Read the model definition and answer for the solid it produces. Units are mm, in the model's axes. A direction names the side the tool comes from. Give positions to 0.01 mm unless a question says otherwise; leave off trailing zeros. Write each loop counter-clockwise with the first axis right and the second up, starting at its lowest first coordinate (ties: lowest second). Pieces come first, ordered by that corner, then holes. Notation, with made-up numbers: (75.5, -23.5) - (86.5, -23.5) arc R16 ccw to (86.5, -0.5) - close; hole circle Ø11 at (55, 60.5). An arc over 180 degrees is marked (long way). Answer as a JSON object with one key per item and string values. Group by question number.
```python
from build123d import *

# Parameters (mm, degrees)
F0_W     = 119
F0_H     = 119
F1_DEPTH = 2.2
F3_DEPTH = 30
F4_R     = 38
F5_DEPTH = 30
F6_T     = -2.2
F7_DEPTH = 1


with BuildPart() as f1:
    # F0 (on Top) → F1 (new body)
    with BuildSketch(Plane.XY):
        Rectangle(F0_W, F0_H)
    extrude(amount=F1_DEPTH)

    # F7 (add): a face of the model
    f7_faces = [f1.faces().sort_by_distance(p)[0] for p in [
        (0, 0, 2.2),
    ]]


with BuildPart() as f3:
    # F2 (on face) → F3 (new body)
    with BuildSketch(Plane.XY.offset(2.2)):
        with BuildLine():
            ThreePointArc((-54.5, 0), (-40.3438347211, -41.7435124756), (0, -59.5))
            ThreePointArc((0, -59.5), (59.5, 0), (0, 59.5))
            Line((0, 59.5), (-59.5, 59.5))
            Line((-59.5, 59.5), (-59.5, 0))
            Line((-59.5, 0), (-54.5, 0))
        make_face()
    extrude(amount=F3_DEPTH)

    # F4 (on face) → F5 (cut, through all)
    with BuildSketch(Plane.XY.offset(32.2)):
        Circle(F4_R)
    extrude(amount=-F5_DEPTH, mode=Mode.SUBTRACT)

    # F6
    f6_openings = [f3.faces().sort_by_distance(p)[0] for p in [
        (-59.5, 29.75, 17.2),
    ]]
    offset(amount=F6_T, openings=f6_openings, kind=Kind.INTERSECTION)


with BuildPart() as f1_1:
    add(f1.part)

    add(f3.part)  # F7 merges F3
    extrude(f7_faces, amount=-F7_DEPTH)


solid = f1_1.part
```
1) Which of the six approach directions +Z, -Z, +X, -X, +Y, -Y give full straight-line access (tool end or side, diameter ignored) to faces 5 (the flat face through (-56, 2.2, 17)), 6 (the cylindrical face through (57.286, -1.26, 17.021)), 7 (the flat face through (45, 48, 2.2)), 8 (the flat face through (47, -47, 2.2)), 9 (the flat face through (-1, 1, 2.2))?
2) Find section D-D, the plane x = -15. Write down the section's boundary in (y, z), and give its area (3 significant figures).
3) For a pull along X with two mould halves and no side action, classify faces 1 (the cylindrical face through (-39.93, -38.89, 17.02)), 2 (the cylindrical face through (17.535, -33.713, 17.41)), 3 (the flat face through (-1, 1, 0)), 4 (the cylindrical face through (-40.77, -41.27, 16.99)) as released by +X, released by -X, zero draft, split by the parting line, or undercut.
4) Find section B-B, the plane x = 21.5. Write down the section's boundary in (y, z).
5) Flat-ended cylindrical pins translate along their axes: pin 1 Ø10 at (y, z) = (10.5, 10.5) entering from +X; pin 2 Ø3 at (y, z) = (-45, 9) entering from +X; pin 3 Ø2.5 at (x, z) = (-57.5, 10.5) entering from -Y. Find the tip coordinate at first contact, or state that the pin passes through.
6) Find the intervals of material crossed by line 1 (Z direction, x = 22, y = 39); line 2 (X direction, y = -6.5, z = 14.5); line 3 (Y direction, x = 12, z = 15), in increasing order. Write a range as [from, to].
7) Find section A-A, the plane z = 17. Write down the section's boundary in (x, y), and give its area (3 significant figures).
8) Find section C-C, the plane y = -42.5. Write down the section's boundary in (x, z), and give its area (3 significant figures).
Values follow:
{
 "1": {"face 5": "-X", "face 6": "none", "face 7": "+Z, +X, +Y", "face 8": "+Z, +X, -Y", "face 9": "+Z"},
 "2": {"outline": "(-59.5, 0) - (59.5, 0) - (59.5, 32.2) - (34.91, 32.2) - (34.91, 2.2) - (-34.91, 2.2) - (-34.91, 32.2) - (-57.4, 32.2) - (-57.4, 2.2) - (-59.5, 2.2) - close; hole (-55.11, 4.4) - (-37.3, 4.4) - (-37.3, 30) - (-55.11, 30) - close; hole (37.3, 4.4) - (57.3, 4.4) - (57.3, 30) - (37.3, 30) - close", "area": "706 mm2"},
 "3": {"face 1": "undercut", "face 2": "undercut", "face 3": "zero draft", "face 4": "released by -X"},
 "4": {"outline": "(-59.5, 0) - (59.5, 0) - (59.5, 2.2) - (55.48, 2.2) - (55.48, 32.2) - (31.33, 32.2) - (31.33, 2.2) - (-31.33, 2.2) - (-31.33, 32.2) - (-55.48, 32.2) - (-55.48, 2.2) - (-59.5, 2.2) - close; hole (-53.11, 4.4) - (-33.97, 4.4) - (-33.97, 30) - (-53.11, 30) - close; hole (33.97, 4.4) - (53.11, 4.4) - (53.11, 30) - (33.97, 30) - close"},
 "5": {"pin 1": "stops at x = 59.25", "pin 2": "stops at x = 40.6", "pin 3": "stops at y = 0"},
 "6": {"line 1": "z = [0, 4.4], [30, 32.2]", "line 2": "x = [-54.68, -52.48], [-39.67, -37.44], [37.44, 39.67], [56.93, 59.14]", "line 3": "y = [-58.28, -56.03], [-38.37, -36.06], [36.06, 38.37], [56.03, 58.28]"},
 "7": {"outline": "(-59.5, 0) - (-54.5, 0) arc R54.71 ccw to (0, -59.5) arc R59.5 ccw to (0, 59.5) - (-59.5, 59.5) - (-59.5, 57.3) - (0, 57.3) arc R57.3 cw to (0, -57.3) arc R52.51 cw to (-52.04, 2.2) - (-59.5, 2.2) - close; circle Ø80.4 at (0, 0); hole circle Ø76 at (0, 0)", "area": "1,290 mm2"},
 "8": {"outline": "(-59.5, 0) - (59.5, 0) - (59.5, 2.2) - (41.64, 2.2) - (41.64, 32.2) - (-39.64, 32.2) - (-39.64, 2.2) - (-59.5, 2.2) - close; hole (-36.54, 4.4) - (38.43, 4.4) - (38.43, 30) - (-36.54, 30) - close", "area": "781 mm2"}
}
